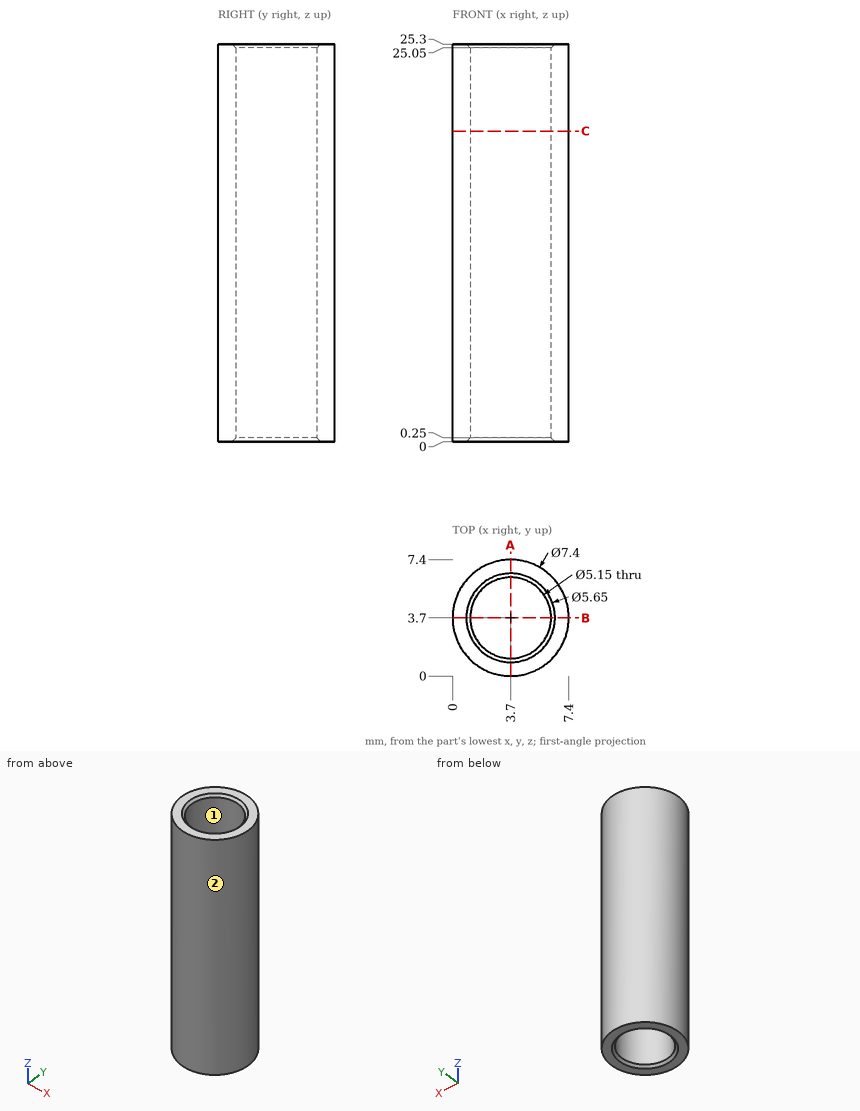
The figure shows three views and two pictorial views of one solid part (mm, origin at its lowest corner). Answer the questions. Coordinates: 2 decimals unless noted, no trailing zeros. Loops run counter-clockwise (first coordinate to the right, second up) from the corner with the lowest first, then second, coordinate; pieces in that order, holes last. Notation, with made-up numbers: (10, 18) -> (55, 18) arc R28 ccw to (55, 46) -> close; hole circle Ø1 at (-13.75, -40). An arc over 180 degrees is marked (long way). Return JSON: item names as keys, results as strings. Group by question number.
(1) Given pin 1 Ø1.5 at (x, z) = (6.5, 20) entering from +Y, flat-ended and moving along its own axis, determine where the tip first touches the part or whether it passes through.
(2) Determine the mould class of the marked faces 1 and 2 for opening direction Y: released by +Y, released by -Y, zero draft, split by the parting line, or undercut.
(3) A cutting plane is placed at A-A on x = 3.7. Write down the section's boundary in (y, z) (3 decimals).
(4) A cutting plane is placed at C-C on z = 19.75. Write down the section's boundary in (x, y) (3 decimals).
(5) Find the intervals of material crossed by probe 1 along Y at (x, z) = (3.7, 8) (3 decimals); probe 2 along X at (y, z) = (3, 24.25); probe 3 along Y at (x, z) = (4.75, 13), in increasing order. Write a range as from..to.
The answers:
{
 "1": {"pin 1": "stops at y = 6.78"},
 "2": {"face 1": "undercut", "face 2": "split by the parting line"},
 "3": {"outline": "(0, 0) -> (0.875, 0) -> (1.125, 0.25) -> (1.125, 25.05) -> (0.875, 25.3) -> (0, 25.3) -> close; (6.275, 0.25) -> (6.525, 0) -> (7.4, 0) -> (7.4, 25.3) -> (6.525, 25.3) -> (6.275, 25.05) -> close"},
 "4": {"outline": "circle Ø7.4 at (3.7, 3.7); hole circle Ø5.15 at (3.7, 3.7)"},
 "5": {"probe 1": "y = 0..1.125, 6.275..7.4", "probe 2": "x = 0.07..1.22, 6.18..7.33", "probe 3": "y = 0.15..1.35, 6.05..7.25"}
}
